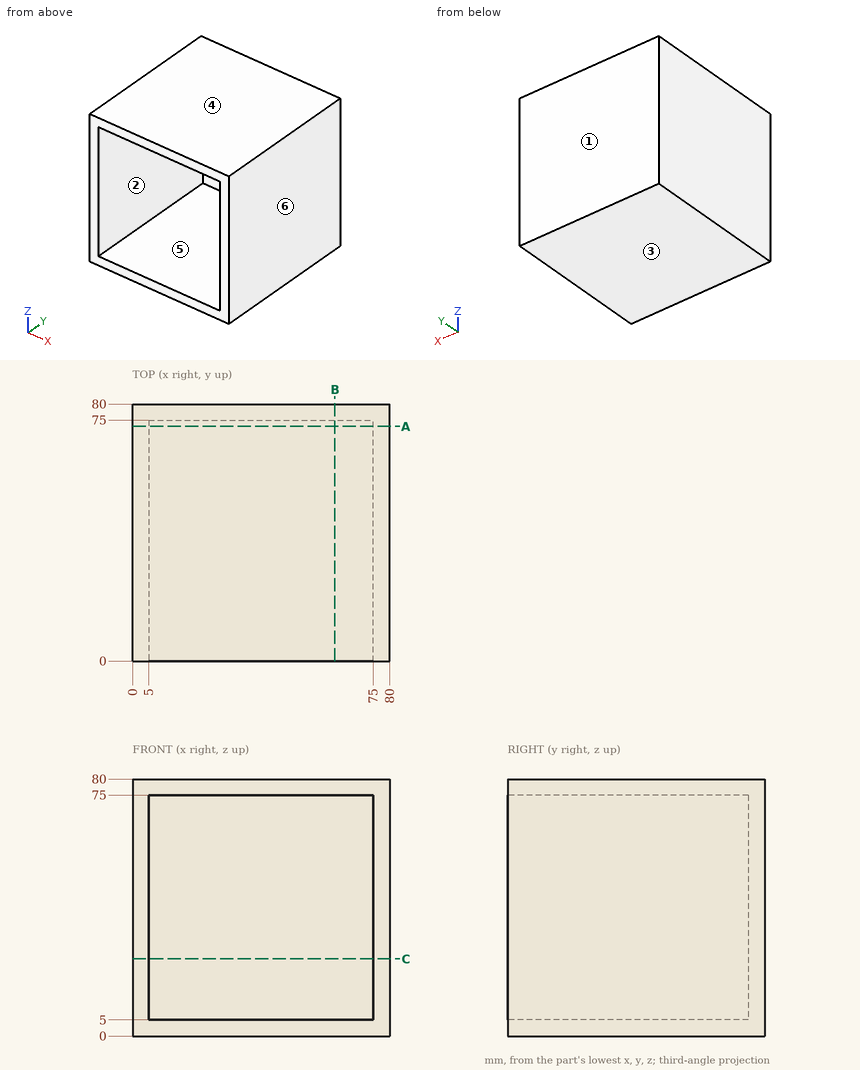
Drawing for the job (mm, zero at the part's lowest x, y, z). A direction names the side the tool comes from. Round coordinates to 2 decimals unless told otherwise and drop trailing zeros. Write each loop counter-clockwise with the first axis right and the second up, starting at its lowest first coordinate (ties: lowest second). Pieces come first, ordered by that corner, then holes. Notation, with made-up numbers: (24, -23.5) - (63, -23.5) arc R6 cw to (63, -13.5) - close; hole circle Ø1 at (-15, -29.5). An arc over 180 degrees is marked (long way). Write item = value, one per line. Start each with the question number.
Q1. Band-saw the part on A-A (y = 73). Give the cut face in (x, z).
Q2. Mould opens along Z. For the marked faces 3, 4, 5 and 6 say: pulls with the +Z half, pulls with the -Z half, needs draft (parallel to the pull), parting line crosses it, or undercut.
Q3. Band-saw the part on C-C (z = 24). Give the cut face in (x, y), then the cut area to 3 significant figures.
Q4. Drop flat-ended pins along their axis: pin 1 (4 mm diameter, centred on x = 35, z = 47, fed in from -Y); pin 2 (1.5 mm diameter, centred on y = 27.5, z = 10, fed in from -X). Give the stop position or say it passes through.
Q5. Which spindle directions (+Z, -Z, +X, -X, +Y, -Y) get a long thin tool onto all of the face, cutting with end or side? Do the marked faces 1 and 2. Say none if no direction does.
Q6. Band-saw the part on B-B (x = 63). Give the cut face in (y, z), then the cut area to 3 significant figures.
Q7. Probe L1, parallel to X at y = 43, z = 66.5; L2, parallel to Y at x = 72, z = 58. List the from-to ranges inside material, lowest first. Write a range as from..to.
Answers below:
q1.outline = (0, 0) - (80, 0) - (80, 80) - (0, 80) - close; hole (5, 5) - (75, 5) - (75, 75) - (5, 75) - close
q2.face_3 = pulls with the -Z half
q2.face_4 = pulls with the +Z half
q2.face_5 = undercut
q2.face_6 = needs draft
q3.outline = (0, 0) - (5, 0) - (5, 75) - (75, 75) - (75, 0) - (80, 0) - (80, 80) - (0, 80) - close
q3.area = 1,150 mm2
q4.pin_1 = 75
q4.pin_2 = 0
q5.face_1 = +Z, -Z, +X, -X, +Y
q5.face_2 = -Y
q6.outline = (0, 0) - (80, 0) - (80, 80) - (0, 80) - (0, 75) - (75, 75) - (75, 5) - (0, 5) - close
q6.area = 1,150 mm2
q7.L1 = 0..5, 75..80
q7.L2 = 75..80
